from build123d import *

# Parameters (mm, degrees)
F1_DEPTH = 12.25
F5_DEPTH = 11.25
F6_R     = 2.5
F7_DEPTH = 2.9
F8_R     = 1
F9_DEPTH = 18.901
F10_R    = 1


with BuildPart() as f1:
    # F0 (on Right) → F1 (new body)
    with BuildSketch(Plane.YZ):
        Polygon((-5.05, -11.5), (12.25, -11.5), (12.25, 11.5), (-5.05, 11.5), (-5.05, 16), (-6.65, 16), (-6.65, 11.5), (-12.25, 11.5), (-12.25, -2.3), (-9.8814561435, -11.5), (-6.65, -11.5), (-6.65, -16), (-5.05, -16), align=None)
    extrude(amount=F1_DEPTH)

    # F4 (on offset) → F5 (join, through all)
    with BuildSketch(Plane.YZ.offset(11.75)):
        Polygon((-10.0745439579, -10.75), (-12.25, -2.3), (-12.25, -9.1), align=None)
    extrude(amount=-F5_DEPTH)

    # F6 (on face) → F7 (join)
    with BuildSketch(Plane.XZ.offset(12.25)):
        with Locations((6.125, 6.1)):
            Circle(F6_R)
    extrude(amount=F7_DEPTH)

    # F8 (on face) → F9 (cut, through all)
    with BuildSketch(Plane.XZ.offset(6.65)):
        with Locations((6.125, 13.75)):
            Circle(F8_R)
        with Locations((6.125, -13.75)):
            Circle(F8_R)
    extrude(amount=-F9_DEPTH, mode=Mode.SUBTRACT)

    # F10
    f10_edges = [f1.edges().sort_by_distance(p)[0] for p in [
        (12.25, 3.6, 11.5),
        (12.25, -9.45, 11.5),
        (12.25, 3.6, -11.5),
        (12.25, -8.265728, -11.5),
        (0, -8.265728, -11.5),
        (0, 3.6, -11.5),
        (0, 3.6, 11.5),
        (0, -9.45, 11.5),
        (0, -5.85, 16),
        (12.25, -5.85, 16),
        (0, -5.85, -16),
        (12.25, -5.85, -16),
    ]]
    fillet(f10_edges, radius=F10_R)


solid = f1.part
Here's how the part is built. I have some questions about the finished solid (model axes, mm). A direction names the side the tool comes from. Give positions to 0.01 mm unless a question says otherwise; leave off trailing zeros. Order: outer loops, then holes, each group sorted by start corner. A loop starts at its lowest first (then second) coordinate and runs counter-clockwise, first axis right, second up. Notation, with made-up numbers: (19, 79.5) -> (42, 79.5) arc R30 cw to (42, 102.5) -> close; hole circle Ø11 at (59, -34). An arc over 180 degrees is marked (long way). Use a Markdown table: item, result. Add a question column.
Item 1: Imagine slicing it at C-C on x = 2.25. Please give me the cut outline in (y, z), plus the area to 3 significant figures.
Item 2: Imagine slicing it at A-A on z = -13.75. Please give me the cut outline in (x, y) (3 decimals), plus the area to 3 significant figures.
Item 3: I need wall thicknesses on line 1 (Y direction, x = 11, z = -8.5); line 2 (Z direction, x = 6.5, y = -7); line 3 (Y direction, x = 3.75, z = -11). Which ranges of each line are inside material? Lowest first, please.
Item 4: Imagine slicing it at B-B on y = -0.5. Please give me the cut outline in (x, z).
Item 5: Imagine slicing it at D-D on z = 6.1. Please give me the cut outline in (x, y) (3 decimals), plus the area to 3 significant figures.
Item 6: For faces 1 (the face through (0.5, -12, -7)), 2 (the face through (0, 0, 0)), 3 (the face through (0.285, 3.479, 11.199)), 4 (the face through (0.301, 3.721, -11.215)), 5 (the face through (11.949, 3.721, -11.215)), which set-ups out of +Z, -Z, +X, -X, +Y, -Y let a thin tool reach every point of the face, with its end or its side?
Item 7: If we mould it in two halves opening along Z, with no side actions, what happens to faces 6 (the face through (5.908, -5.861, -14.726)), 7 (the face through (6, -9, 11.5)), 8 (the face through (11.965, -8.37, -11.199))? For each: pulls with the +Z half, pulls with the -Z half, needs draft (parallel to the pull), parting line crosses it, or undercut.
Item 8: Will these pins go through, and if not, where does the flat tip stop? pin 1 (1 mm diameter, centred on x = 3, z = -6.5, fed in from -Y); pin 2 (1 mm diameter, centred on x = 2.5, z = -10, fed in from -Y); pin 3 (2.5 mm diameter, centred on x = 6.125, z = -13.75, fed in from -Y).
Data:
| question | item | result |
|---|---|---|
| 1 | outline | (-12.25, -9.1) -> (-10.07, -10.75) -> (-9.88, -11.5) -> (-6.65, -11.5) -> (-6.65, -16) -> (-5.05, -16) -> (-5.05, -11.5) -> (12.25, -11.5) -> (12.25, 11.5) -> (-5.05, 11.5) -> (-5.05, 16) -> (-6.65, 16) -> (-6.65, 11.5) -> (-12.25, 11.5) -> close |
| 1 | area | 574 mm² |
| 2 | outline | (0, -6.65) -> (5.125, -6.65) -> (5.125, -5.05) -> (0, -5.05) -> close; (7.125, -6.65) -> (12.25, -6.65) -> (12.25, -5.05) -> (7.125, -5.05) -> close |
| 2 | area | 16.4 mm² |
| 3 | line 1 | y = -12.25 to 12.25 |
| 3 | line 2 | z = -11.5 to 11.5 |
| 3 | line 3 | y = -10.01 to 12.25 |
| 4 | outline | (0, -10.5) arc R1 ccw to (1, -11.5) -> (11.25, -11.5) arc R1 ccw to (12.25, -10.5) -> (12.25, 10.5) arc R1 ccw to (11.25, 11.5) -> (1, 11.5) arc R1 ccw to (0, 10.5) -> close |
| 5 | outline | (0, -12.25) -> (3.625, -12.25) -> (3.625, -15.15) -> (8.625, -15.15) -> (8.625, -12.25) -> (12.25, -12.25) -> (12.25, 12.25) -> (0, 12.25) -> close |
| 5 | area | 315 mm² |
| 6 | face 1 | -Z, -X, -Y |
| 6 | face 2 | +Z, -Z, -X, +Y, -Y |
| 6 | face 3 | +Z, -X, +Y |
| 6 | face 4 | -Z, -X, +Y |
| 6 | face 5 | -Z, +X, +Y |
| 7 | face 6 | undercut |
| 7 | face 7 | pulls with the +Z half |
| 7 | face 8 | pulls with the -Z half |
| 8 | pin 1 | stops at y = -12.25 |
| 8 | pin 2 | stops at y = -11.72 |
| 8 | pin 3 | stops at y = -6.65 |
